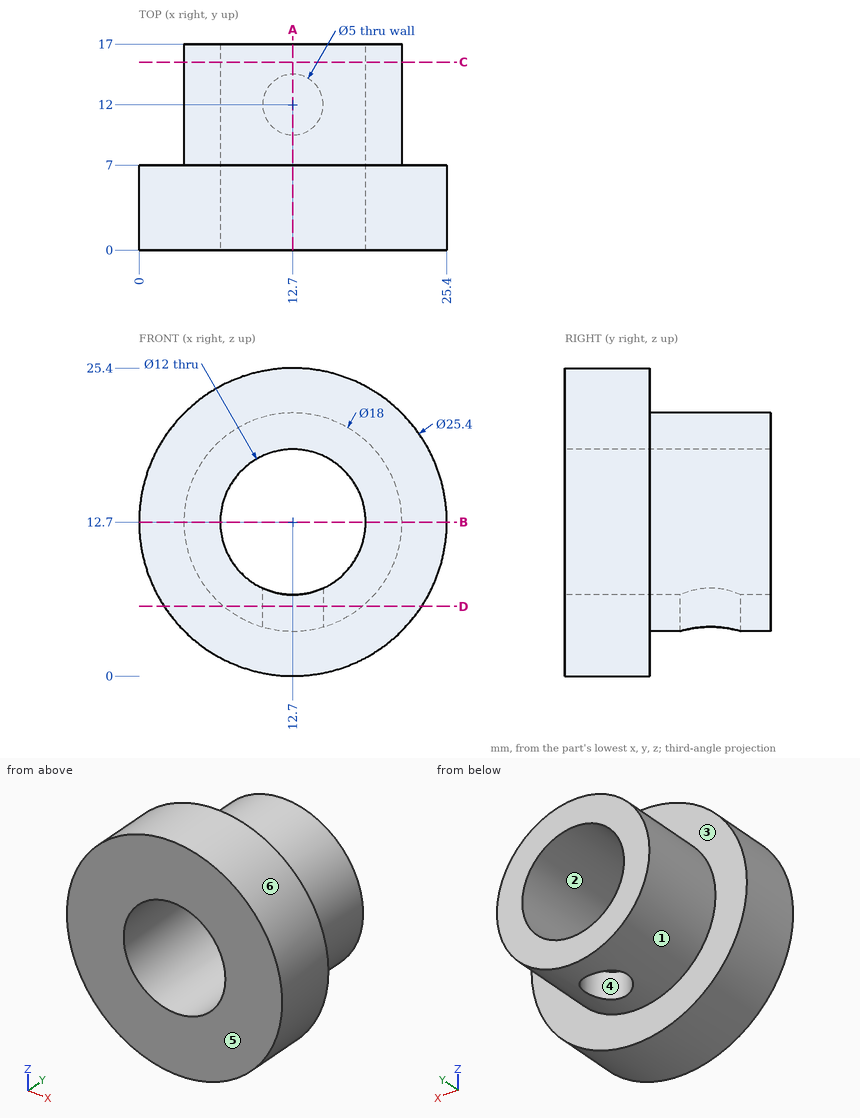
Study the drawing (mm; zero at the part's minimum x, y, z) and answer. A direction names the side the tool comes from. Give positions to 0.01 mm unless a question says otherwise; leave off trailing zeros. Write each loop counter-clockwise with the first axis right and the second up, starting at its lowest first coordinate (ties: lowest second). Pieces come first, ordered by that corner, then holes. Notation, with made-up numbers: (30, -9) -> (66, -9) arc R6 ccw to (66, 2) -> close; hole circle Ø2 at (42.5, -35). An arc over 180 degrees is marked (long way). Answer as a JSON object with one key per item and string values. Group by question number.
1) A tool of negligible diameter and unlimited length cuts with its end or side. For the marked faces 1 and 2, from which of +Z, -Z, +X, -X, +Y, -Y can it reach the whole face along a straight path? Write none if from no direction.
2) Find section A-A (x = 12.7). Write down the section's boundary in (y, z).
3) Find section B-B (z = 12.7). Write down the section's boundary in (x, y), and give its area (3 significant figures).
4) Consider L1, parallel to Y at x = 9, z = 24; L2, parallel to Z at x = 16, y = 2; L3, parallel to Z at x = 12, y = 9.5. Determine where each line is inside the solid, lowest interval first. Write a range as from..to.
5) Find section C-C (y = 15.5). Write down the section's boundary in (x, z), and give its area (3 significant figures).
6) Find section D-D (z = 5.75). Write down the section's boundary in (x, y).
7) The mould has two halves that part along Y. Classify the marked faces 3, 4, 5 and 6: +Y half, -Y half, draft (parallel to the pull), parting line (faces both ways), or undercut.
8) Each of these flat-tipped pins is pushed along its axis until it touches: P1, Ø4, axis at x = 19, y = 8.5, coming from the +Z side; P2, Ø1, axis at x = 6.5, y = 6, coming from the +Z side; P3, Ø7, axis at x = 12.7, z = 12.7, coming from the +Y side; P4, Ø3, axis at x = 12.7, y = 12, coming from the -Z side. Where does it stop, or does it pass through?
Values follow:
{
 "1": {"face 1": "+Y", "face 2": "+Y, -Y"},
 "2": {"outline": "(0, 0) -> (7, 0) -> (7, 3.7) -> (9.5, 3.7) -> (9.5, 6.7) -> (0, 6.7) -> close; (0, 18.7) -> (17, 18.7) -> (17, 21.7) -> (7, 21.7) -> (7, 25.4) -> (0, 25.4) -> close; (14.5, 3.7) -> (17, 3.7) -> (17, 6.7) -> (14.5, 6.7) -> close"},
 "3": {"outline": "(0, 0) -> (6.7, 0) -> (6.7, 17) -> (3.7, 17) -> (3.7, 7) -> (0, 7) -> close; (18.7, 0) -> (25.4, 0) -> (25.4, 7) -> (21.7, 7) -> (21.7, 17) -> (18.7, 17) -> close", "area": "154 mm2"},
 "4": {"L1": "y = 0..7", "L2": "z = 0.44..7.69, 17.71..24.96", "L3": "z = 3.73..6.74, 18.66..21.67"},
 "5": {"outline": "circle Ø18 at (12.7, 12.7); hole circle Ø12 at (12.7, 12.7)", "area": "141 mm2"},
 "6": {"outline": "(2.07, 0) -> (23.33, 0) -> (23.33, 7) -> (18.42, 7) -> (18.42, 17) -> (6.98, 17) -> (6.98, 7) -> (2.07, 7) -> close; hole circle Ø5 at (12.7, 12)"},
 "7": {"face 3": "+Y half", "face 4": "undercut", "face 5": "-Y half", "face 6": "draft"},
 "8": {"P1": "stops at z = 24.38", "P2": "stops at z = 24.05", "P3": "passes through", "P4": "stops at z = 18.51"}
}
